from build123d import *

# Parameters (mm, degrees)
EXTRUDE_1_DEPTH     = 5
SKETCH_2_R          = 1.5
CUT_EXTRUDE_1_DEPTH = 21
FILLET_1_R          = 2.5


with BuildPart() as part:
    # 草图1 → 凸台-拉伸1 (new body)
    with BuildSketch(Plane(origin=(0, 0, 0), x_dir=(0, 0, -1), z_dir=(1, 0, 0))):
        Polygon((-2.5, 20), (-2.5, 7), (2.5, 7), (2.5, 20), (9, 20), (9, -20), (2.5, -20), (2.5, -7), (-2.5, -7), (-2.5, -20), (-9, -20), (-9, 20), align=None)
    extrude(amount=EXTRUDE_1_DEPTH)

    # 草图2 → 切除-拉伸1 (cut)
    with BuildSketch(Plane.XY.offset(9)):
        with Locations((2.5, 12.5)):
            Circle(SKETCH_2_R)
        with Locations(Location((2.5, -12.5, 0), (0, 0, 270))):
            Circle(SKETCH_2_R)
    extrude(amount=-CUT_EXTRUDE_1_DEPTH, mode=Mode.SUBTRACT)

    # 圆角1
    fillet_1_edges = [part.edges().sort_by_distance(p)[0] for p in [
        (2.5, 7, -2.5),
        (2.5, 7, 2.5),
        (2.5, -7, -2.5),
        (2.5, -7, 2.5),
    ]]
    fillet(fillet_1_edges, radius=FILLET_1_R - 0.0001)  # a hair under: the kernel refuses the full size


solid = part.part
Input: part model. Units: mm. Frame: model coordinates. A direction names the side the tool comes from. Coordinates: 2 decimals unless noted, no trailing zeros. Write each loop counter-clockwise with the first axis right and the second up, starting at its lowest first coordinate (ties: lowest second). Pieces come first, ordered by that corner, then holes. Notation, with made-up numbers: M 23.25,31.25 L 43.25,31.25 A26 ccw 43.25,52.25 Z; hole C 15,76 d10. An arc over 180 degrees is marked long. Answer as a JSON object with one key per item and string values. Group by question number.
(1) Section D-D on z = -7.25. Output: boundary loops of the cut face in (x, y).
(2) Section A-A on y = -17. Output: boundary loops of the cut face in (x, z), plus the area to 3 significant figures.
(3) Ray query, line 1 along Y through (x, z) = (2.35, -8.5); line 2 along Z through (x, y) = (3.8, 13.5); line 3 along X through (y, z) = (-12.5, -5). Return the intervals inside material, ascending. Write a range as [from, to].
(4) Set-up query: faces 5 (the face through (2, -15, -2.5)), 6 (the face through (3, 8, -2)), 7 (the face through (2, 20, -6)). Return all of +Z, -Z, +X, -X, +Y, -Y with unobstructed straight access to the full face (end or side cutting, diameter ignored); none if empty.
(5) Section B-B on x = 1.6. Give the number of separate pieces and of enclosed holes in the cut face, plus the area to 3 significant figures.
(6) Section C-C on y = -12.5. Output: boundary loops of the cut face in (x, z), plus the area to 3 significant figures.
(7) Mould query, pull axis Z, two halves, no side actions, for faces 1 (the face through (1.036, -12.175, 5.796)), 2 (the face through (2, 15, -2.5)), 3 (the face through (2, 0, -9)), 4 (the face through (3, 8, 2)). Classes: pulls with the +Z half, pulls with the -Z half, needs draft (parallel to the pull), parting line crosses it, or undercut.
(8) Contact query for a flat-ended pin moving along its axis: P1, Ø2.5, axis at x = 2.5, y = 12.5, coming from the -Z side. Output: stop coordinate, or through.
Result set:
{
 "1": {"outline": "M 0,-20 L 5,-20 L 5,20 L 0,20 Z; hole C 2.5,-12.5 d3; hole C 2.5,12.5 d3"},
 "2": {"outline": "M 0,-9 L 5,-9 L 5,-2.5 L 0,-2.5 Z; M 0,2.5 L 5,2.5 L 5,9 L 0,9 Z", "area": "65.0 mm2"},
 "3": {"line 1": "y = [-20, -13.99], [-11.01, 11.01], [13.99, 20]", "line 2": "z = [-9, -2.5], [2.5, 9]", "line 3": "x = [0, 1], [4, 5]"},
 "4": {"face 5": "+X, -X, -Y", "face 6": "+X, -X, +Y", "face 7": "+Z, -Z, +X, -X, +Y"},
 "5": {"separate pieces": "5", "enclosed holes": "0", "area": "533 mm2"},
 "6": {"outline": "M 0,-9 L 1,-9 L 1,-2.5 L 0,-2.5 Z; M 0,2.5 L 1,2.5 L 1,9 L 0,9 Z; M 4,-9 L 5,-9 L 5,-2.5 L 4,-2.5 Z; M 4,2.5 L 5,2.5 L 5,9 L 4,9 Z", "area": "26.0 mm2"},
 "7": {"face 1": "needs draft", "face 2": "undercut", "face 3": "pulls with the -Z half", "face 4": "undercut"},
 "8": {"P1": "passes through"}
}
